Solid Edge part; units mm, degrees
sketch "Sketch1" plane through (0, 0, 0) normal (0, -1, 0) x (1, 0, 0)
  line L0 (-60, 37) -> (-15, 0)
  line L1 (-15, 0) -> (15, 0)
  line L2 (15, 0) -> (60, 37)
  line L3 (60, 37) -> (-60, 37)
  dimension "D1" = 15
  dimension "D2" = 60
  dimension "D3" = 60
extrude "Protrusion1" add sketch "Sketch1" against normal blind 40
sketch "Sketch2" plane through (0, 40, 18.5) normal (0, 1, 0) x (-1, 0, 0)
  line L0 (-8, -18.5) -> (8, -18.5)
  line L1 (8, -18.5) -> (8, 11.5)
  line L2 (8, 11.5) -> (-8, 11.5)
  line L3 (-8, 11.5) -> (-8, -18.5)
  line L4 (-40.4647, 11.5) -> (-15, -9.4376)
  line L5 (-15, -9.4376) -> (-15, 11.5)
  line L6 (-15, 11.5) -> (-40.4647, 11.5)
  line L7 (40.4647, 11.5) -> (15, -9.4376)
  line L8 (15, -9.4376) -> (15, 11.5)
  line L9 (15, 11.5) -> (40.4647, 11.5)
  dimension "D1" = 8
extrude "ExtrudedCutout_1" cut sketch "Sketch2" against normal blind 33
sketch "Sketch3" plane through (0, 7, 15) normal (0, 1, 0) x (-1, 0, 0)
  circle A0 centre (0, -11.5) radius 1.7
  circle A1 centre (0, 4.5) radius 1.7
extrude "Cutout1" cut sketch "Sketch3" against normal through all
sketch "Sketch4" plane through (0, 0, 0) normal (1, 0, 0) x (0, 1, 0)
  line L0 (7, 0) -> (40, 30)
extrude "Cutout2" cut sketch "Sketch4" against normal through all and the other way through all material side at (0, 23.5336, 14.963)
sketch "Sketch5" plane through (0, 0, 0) normal (1, 0, 0) x (0, 1, 0)
  line L0 (40, 37) -> (40, 58)
  line L1 (40, 58) -> (33, 58)
  line L2 (33, 58) -> (33, 40)
  arc A0 (30, 37) -> (33, 40) centre (30, 40) ccw
  line L3 (40, 37) -> (30, 37)
  dimension "D1" = 40
  dimension "D2" = 40
extrude "ExtrudedProtrusion_3" add sketch "Sketch5" along normal mid plane 120
fillet "Round_1" radius 3 1 edges at (0, 0, 37)
sketch "Sketch6" plane through (0, 0, 0) normal (0, -1, 0) x (1, 0, 0)
  circle A0 centre (-50, 49) radius 1.7
  circle A1 centre (50, 49) radius 1.7
  dimension "D1" = 50
extrude "Cutout3" cut sketch "Sketch6" against normal through all
properties material "ABS Plastic, medium impact"
Source: CAD feature listing. Evaluate the final solid. Frame: model axes, mm. A direction names the side the tool comes from. Round coordinates to 2 decimals unless told otherwise and drop trailing zeros. Write each loop counter-clockwise with the first axis right and the second up, starting at its lowest first coordinate (ties: lowest second). Pieces come first, ordered by that corner, then holes. Notation, with made-up numbers: (-19, 15) - (19, 15) arc R15 cw to (19, 37) - close; hole circle Ø9 at (47.25, -5.75). An arc over 180 degrees is marked (long way). Use CSV: the item, a comma, the result in double quotes. Start each with the question number.
(1) Set-up query: faces 1 (the face through (0, 7, 15)), 2 (the face through (28, 24, 30)), 3 (the face through (-24.61, 23.27, 14.79)). Return all of +Z, -Z, +X, -X, +Y, -Y with unobstructed straight access to the full face (end or side cutting, diameter ignored); none if empty.
(2) First-contact query: pin 1 Ø1.5 at (x, y) = (-30.5, 11) entering from -Z; pin 2 Ø10 at (y, z) = (12, 22.5) entering from +X; pin 3 Ø14.5 at (x, z) = (-5, 46) entering from -Y; pin 4 Ø12 at (x, z) = (37, 23) entering from -Y. Flat tips, straight axial feed; report the tip coordinate or a pass-through.
(3) Cut plane C-C, the plane y = 4.5. Return loops of the section in (x, z).
(4) Mould query, pull axis X, two halves, no side actions, for faces 4 (the face through (-1, 33, 49)), 5 (the face through (42.18, 15.28, 22.35)), 6 (the face through (-60, 36, 47)), 7 (the face through (-8, 16, 21)). Classes: pulls with the +X half, pulls with the -X half, needs draft (parallel to the pull), parting line crosses it, or undercut.
(5) Cut plane D-D, the plane x = -50. Return loops of the section in (y, z).
(6) Cut plane B-B, the plane z = 49. Return loops of the section in (x, y), and give its area (3 significant figures).
(7) Cut plane A-A, the plane x = 0. Return loops of the section in (y, z).
(8) Material intervals for probe 1 along Z at (x, y) = (0, 5); probe 2 along Z at (x, y) = (-27, 37.5); probe 3 along Z at (x, y) = (-13, 3.5), sorted ascending. Write a range as [from, to].
Geometry says:
1,face 1,"-Z, +Y"
1,face 2,"+Y"
1,face 3,"-Z, +X, -X, +Y"
2,pin 1,"z = 12.13"
2,pin 2,"x = 48.45"
2,pin 3,"y = 32.73"
2,pin 4,"y = 0"
3,outline,"(-60, 37) - (-15, 0) - (15, 0) - (60, 37) - close; hole circle Ø3.4 at (0, 3.5); hole circle Ø3.4 at (0, 19.5)"
4,face 4,"needs draft"
4,face 5,"pulls with the +X half"
4,face 6,"pulls with the -X half"
4,face 7,"undercut"
5,outline,"(0, 28.78) - (38.66, 28.78) - (40, 30) - (40, 47.3) - (33, 47.3) - (33, 40) arc R3 cw to (30, 37) - (3, 37) arc R3 ccw to (0, 34) - close; (33, 50.7) - (40, 50.7) - (40, 58) - (33, 58) - close"
6,outline,"(-60, 33) - (-51.7, 33) - (-51.7, 40) - (-60, 40) - close; (-48.3, 33) - (48.3, 33) - (48.3, 40) - (-48.3, 40) - close; (51.7, 33) - (60, 33) - (60, 40) - (51.7, 40) - close"
6,area,"792 mm²"
7,outline,"(0, 0) - (7, 0) - (7, 1.8) - (0, 1.8) - close; (0, 5.2) - (7, 5.2) - (7, 17.8) - (0, 17.8) - close; (0, 21.2) - (7, 21.2) - (7, 30) - (40, 30) - (40, 58) - (33, 58) - (33, 40) arc R3 cw to (30, 37) - (3, 37) arc R3 ccw to (0, 34) - close"
8,probe 1,"[0, 1.8], [5.2, 17.8], [21.2, 37]"
8,probe 2,"[30, 58]"
8,probe 3,"[0, 37]"
